```python
from build123d import *

# Parameters (mm, degrees)
SKETCH_1_R          = 32.5
EXTRUDE_1_DEPTH     = 36
SKETCH_2_R          = 38.5
EXTRUDE_2_DEPTH     = 82
SKETCH_3_R          = 41
EXTRUDE_3_DEPTH     = 12
SKETCH_4_R          = 35
EXTRUDE_4_DEPTH     = 76
SKETCH_5_R          = 32.5
EXTRUDE_5_DEPTH     = 64
SKETCH_6_R          = 31
EXTRUDE_6_DEPTH     = 50
SKETCH_7_R          = 27.5
EXTRUDE_7_DEPTH     = 82
FILLET_1_R          = 2
FILLET_2_R          = 1.6
CHAMFER_1_SIZE      = 2
CUT_EXTRUDE_1_DEPTH = 29


with BuildPart() as part:
    # 草图1 → 凸台-拉伸1 (new body)
    with BuildSketch(Plane.XY):
        Circle(SKETCH_1_R)
    extrude(amount=EXTRUDE_1_DEPTH)

    # 草图2 → 凸台-拉伸2 (add)
    with BuildSketch(Plane.XY.offset(36)):
        Circle(SKETCH_2_R)
    extrude(amount=EXTRUDE_2_DEPTH)

    # 草图3 → 凸台-拉伸3 (add)
    with BuildSketch(Plane.XY.offset(118)):
        Circle(SKETCH_3_R)
    extrude(amount=EXTRUDE_3_DEPTH)

    # 草图4 → 凸台-拉伸4 (add)
    with BuildSketch(Plane.XY.offset(130)):
        Circle(SKETCH_4_R)
    extrude(amount=EXTRUDE_4_DEPTH)

    # 草图5 → 凸台-拉伸5 (add)
    with BuildSketch(Plane.XY.offset(206)):
        Circle(SKETCH_5_R)
    extrude(amount=EXTRUDE_5_DEPTH)

    # 草图6 → 凸台-拉伸6 (add)
    with BuildSketch(Plane.XY.offset(270)):
        Circle(SKETCH_6_R)
    extrude(amount=EXTRUDE_6_DEPTH)

    # 草图7 → 凸台-拉伸7 (add)
    with BuildSketch(Plane.XY.offset(320)):
        Circle(SKETCH_7_R)
    extrude(amount=EXTRUDE_7_DEPTH)

    # 圆角1
    fillet_1_edges = [part.edges().sort_by_distance(p)[0] for p in [
        (-35, 0, 130),
        (-32.5, 0, 206),
    ]]
    fillet(fillet_1_edges, radius=FILLET_1_R)

    # 圆角2
    # the kernel refuses this fillet: 1.6 mm, written as the material it adds along each edge
    with BuildSketch(Plane(origin=(0, 0, 270), x_dir=(1, 0, 0), z_dir=(0, -1, 0))) as fillet_2_piece_1:
        with BuildLine():
            CenterArc((32.6, 1.596871942), FILLET_2_R, 180, 86.416678302)
            Line((31, 1.596871942), (30.968, 1.596871942))
            Line((30.968, 1.596871942), (30.968, 0))
            Line((30.968, 0), (31, -0.032))
            ThreePointArc((31, -0.032), (31.75, -0.032), (32.498, -0.031937439))
            Line((32.498, -0.031937439), (32.5, 0))
        make_face()
    revolve(axis=Axis((0, 0, 270), (0, 0, 1)))
    with BuildSketch(Plane(origin=(0, 0, 320), x_dir=(1, 0, 0), z_dir=(0, -1, 0))) as fillet_2_piece_2:
        with BuildLine():
            CenterArc((27.5 + FILLET_2_R, FILLET_2_R), FILLET_2_R, 180, 90)
            Line((27.5, FILLET_2_R), (27.5 - FILLET_2_R * 0.02, FILLET_2_R))
            Line((27.5 - FILLET_2_R * 0.02, FILLET_2_R), (27.5 - FILLET_2_R * 0.02, -FILLET_2_R * 0.02))
            Line((27.5 - FILLET_2_R * 0.02, -FILLET_2_R * 0.02), (27.5 + FILLET_2_R, -FILLET_2_R * 0.02))
            Line((27.5 + FILLET_2_R, -FILLET_2_R * 0.02), (27.5 + FILLET_2_R, 0))
        make_face()
    revolve(axis=Axis((0, 0, 320), (0, 0, 1)))

    # 倒角1
    chamfer_1_edges = [part.edges().sort_by_distance(p)[0] for p in [
        (-32.5, 0, 0),
        (-27.5, 0, 402),
    ]]
    chamfer(chamfer_1_edges, length=CHAMFER_1_SIZE)

    # 草图8 → 切除-拉伸1 (cut)
    with BuildSketch(Plane(origin=(27.5, 0, 0), x_dir=(0, 0, -1), z_dir=(1, 0, 0))):
        with BuildLine():
            Line((-189, 10), (-146, 10))
            ThreePointArc((-146, 10), (-136, 0), (-146, -10))
            Line((-146, -10), (-189, -10))
            ThreePointArc((-189, -10), (-199, 0), (-189, 10))
        make_face()
    extrude(amount=CUT_EXTRUDE_1_DEPTH, mode=Mode.SUBTRACT)


solid = part.part
```
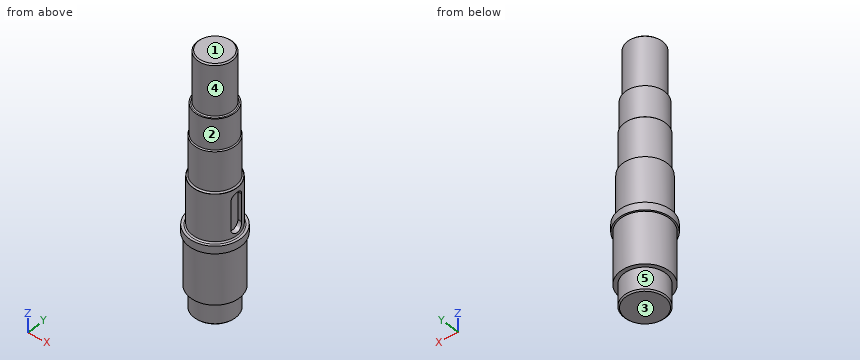
For this review, take the finished solid that the model builds, in its own axes (mm). Face numbers are marked on the shaded views. A direction names the side the tool comes from. Round coordinates to 2 decimals unless told otherwise and drop trailing zeros. Loops run counter-clockwise (first coordinate to the right, second up) from the corner with the lowest first, then second, coordinate; pieces in that order, holes last.
(1) We need section A-A (z = 68). Give the boundary of the cut face in (x, y), plus the area to 3 significant figures.
Returned:
outline: circle Ø77 at (0, 0)
area: 4,660 mm2
(2) Mouldability with a two-part tool opening along Z and no side actions: class the marked faces 1, 2 and 3 as released by +Z, released by -Z, zero draft, split by the parting line, or undercut.
Returned:
face 1: released by +Z
face 2: zero draft
face 3: released by -Z
(3) Tool access review of the marked faces 4 and 5: name each direction out of +Z, -Z, +X, -X, +Y, -Y from which nothing blocks a thin tool from reaching the whole face with its end or side.
Returned:
face 4: +Z
face 5: -Z
(4) Wall thickness on line 1 along Z through (x, y) = (-37, -0.5); line 2 along Z through (x, y) = (22, 28); line 3 along X through (y, z) = (23, 26): over which ranges is each line inside the solid? List them lowest first.
Returned:
line 1: z = 36 to 130
line 2: z = 36 to 130.56
line 3: x = -22.96 to 22.96
(5) Clearance check with flat-ended pins moving along their axes: P1, Ø3, axis at y = 28, z = 106.5, coming from the +X side; P2, Ø3, axis at x = 31, z = 174.5, coming from the -Y side; P3, Ø1.8, axis at x = 31, z = 161.5, coming from the +Y side. State where each tip first meets the part, or that it passes through.
Returned:
P1: stops at x = 27.93
P2: stops at y = -18.83
P3: stops at y = 17.86
